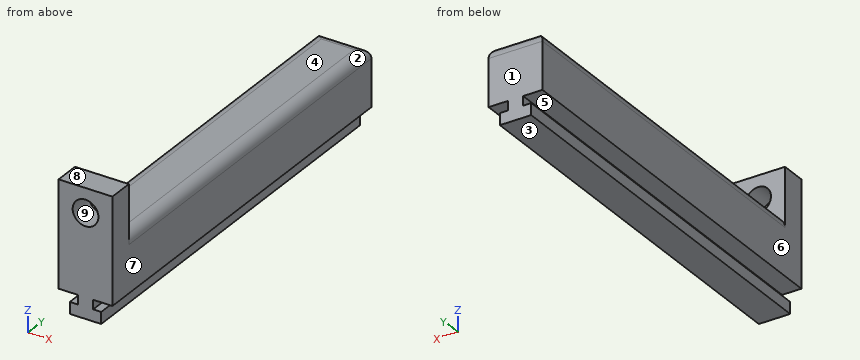
```python
from build123d import *

# Parameters (mm, degrees)
SKETCH1_W               = 8.5
SKETCH1_H               = 20
BOSS_EXTRUDE1_DEPTH     = 63.246
SKETCH2_W               = 8.5
SKETCH2_H               = 7.62
CUT_EXTRUDE1_DEPTH      = 59.246
CUT_EXTRUDE2_DEPTH      = 5.334
CUT_EXTRUDE2_DEPTH_BACK = 79.922
SKETCH5_R               = 2.032
CUT_EXTRUDE3_DEPTH      = 79.922
FILLET1_R               = 1.651


with BuildPart() as part:
    # Sketch1 → Boss-Extrude1 (new body)
    with BuildSketch(Plane(origin=(0, 0, 0), x_dir=(1, 0, 0), z_dir=(0, 1, 0))):
        Rectangle(SKETCH1_W, SKETCH1_H)
    extrude(amount=BOSS_EXTRUDE1_DEPTH)

    # Sketch2 → Cut-Extrude1 (cut)
    with BuildSketch(Plane(origin=(0, 63.246, 0), x_dir=(1, 0, 0), z_dir=(0, 1, 0))):
        with Locations((0, -6.19)):
            Rectangle(SKETCH2_W, SKETCH2_H)
    extrude(amount=-CUT_EXTRUDE1_DEPTH, mode=Mode.SUBTRACT)

    # Sketch4 → Cut-Extrude2 (cut, two sides)
    with BuildSketch(Plane(origin=(0, 63.246, 0), x_dir=(1, 0, 0), z_dir=(0, 1, 0))) as cut_extrude2_sk:
        Polygon((-1.2065, 6.698), (-4.25, 6.698), (-4.25, 10), (-2.4765, 10), (-2.4765, 8.1585), (-1.2065, 8.1585), align=None)
        Polygon((1.2065, 6.698), (4.25, 6.698), (4.25, 10), (2.4765, 10), (2.4765, 8.1585), (1.2065, 8.1585), align=None)
    extrude(amount=CUT_EXTRUDE2_DEPTH, mode=Mode.SUBTRACT)
    extrude(cut_extrude2_sk.sketch, amount=-CUT_EXTRUDE2_DEPTH_BACK, mode=Mode.SUBTRACT)

    # Sketch5 → Cut-Extrude3 (cut)
    with BuildSketch(Plane(origin=(0, 4, 0), x_dir=(1, 0, 0), z_dir=(0, 1, 0))):
        with Locations((0, -6.19)):
            Circle(SKETCH5_R)
    extrude(amount=-CUT_EXTRUDE3_DEPTH, mode=Mode.SUBTRACT)

    # Fillet1
    fillet1_edges = [part.edges().sort_by_distance(p)[0] for p in [
        (4.25, 33.623, 2.38),
        (-4.25, 33.623, 2.38),
        (0, 63.246, 2.38),
    ]]
    fillet(fillet1_edges, radius=FILLET1_R)


solid = part.part
```
Read the model definition and answer for the solid it produces. Units are mm, in the model's axes. Face numbers are marked on the shaded views. A direction names the side the tool comes from. Coordinates: 2 decimals unless noted, no trailing zeros. Loops run counter-clockwise (first coordinate to the right, second up) from the corner with the lowest first, then second, coordinate; pieces in that order, holes last.
(1) The part is cut by section A-A (x = 0). Determine the outline of the cut face in (y, z) (3 decimals), and give its area (3 significant figures).
Solution:
outline: (0, -10) - (63.246, -10) - (63.246, 0.729) arc R1.651 ccw to (61.595, 2.38) - (4, 2.38) - (4, 4.158) - (0, 4.158) - close; (0, 8.222) - (4, 8.222) - (4, 10) - (0, 10) - close
area: 797 mm2
(2) The mould has two halves that part along X. Classify the marked faces 6, 7, 8 and 9: released by +X, released by -X, zero draft, split by the parting line, or undercut.
Solution:
face 6: released by -X
face 7: released by +X
face 8: zero draft
face 9: undercut
(3) A tool of negligible diameter and unlimited length cuts with its end or side. For the marked faces 1, 2, 3, 4 and 5, from which of +Z, -Z, +X, -X, +Y, -Y can it reach the whole face along a straight path? Write none if from no direction.
Solution:
face 1: +Z, -Z, +X, -X, +Y
face 2: +Z, +X, +Y
face 3: -Z, +X, -X, +Y, -Y
face 4: +Z, +X, -X, +Y
face 5: -X, +Y, -Y
(4) The part is cut by section B-B (z = 6.19). Determine the outline of the cut face in (x, y).
Solution:
outline: (-4.25, 0) - (-2.03, 0) - (-2.03, 4) - (-4.25, 4) - close; (2.03, 0) - (4.25, 0) - (4.25, 4) - (2.03, 4) - close
(5) The part is cut by section C-C (y = 44). Determine the outline of the cut face in (x, z), and give its area (3 significant figures).
Solution:
outline: (-4.25, -6.7) - (-1.21, -6.7) - (-1.21, -8.16) - (-2.48, -8.16) - (-2.48, -10) - (2.48, -10) - (2.48, -8.16) - (1.21, -8.16) - (1.21, -6.7) - (4.25, -6.7) - (4.25, 0.73) arc R1.65 ccw to (2.6, 2.38) - (-2.6, 2.38) arc R1.65 ccw to (-4.25, 0.73) - close
area: 88.6 mm2
(6) Flat-ended cylindrical pins translate along their axes: pin 1 Ø1 at (x, z) = (-1, 3.5) entering from +Y; pin 2 Ø1.6 at (x, y) = (0, 36) entering from +Z; pin 3 Ø0.9 at (y, z) = (29, -9) entering from +X. Find the tip coordinate at first contact, or state that the pin passes through.
Solution:
pin 1: stops at y = 4
pin 2: stops at z = 2.38
pin 3: stops at x = 2.48
(7) Consider line 1 along Z through (x, y) = (0, 2.3); line 2 along Z through (x, y) = (-1.75, 6); line 3 along X through (y, z) = (1.2, 6.19). Determine where each line is inside the solid, lowest interval first.
Solution:
line 1: z = -10 to 4.16, 8.22 to 10
line 2: z = -10 to -8.16, -6.7 to 2.38
line 3: x = -4.25 to -2.03, 2.03 to 4.25
(8) The part is cut by section D-D (x = -3.5). Determine the outline of the cut face in (y, z) (3 decimals).
Solution:
outline: (0, -6.698) - (63.246, -6.698) - (63.246, 0.729) arc R1.651 ccw to (62.496, 2.112) - (4, 2.112) - (4, 10) - (0, 10) - close
